Can you work these out from the drawing? Everything is in mm from the part's minimum corner. A direction names the side the tool comes from. Coordinates: 2 decimals unless noted, no trailing zeros. Loops run counter-clockwise (first coordinate to the right, second up) from the corner with the lowest first, then second, coordinate; pieces in that order, holes last.
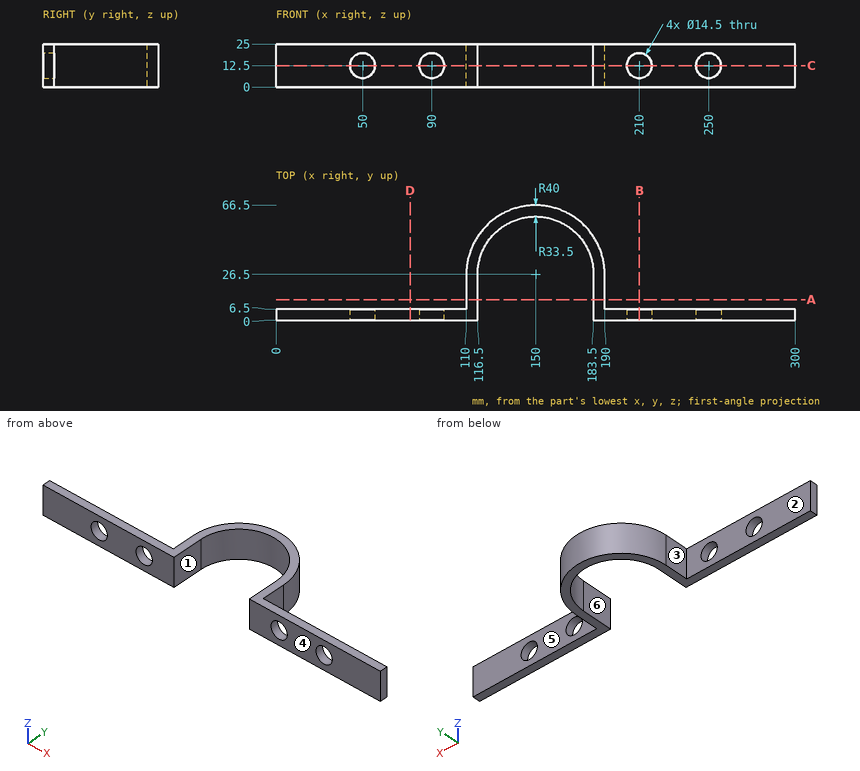
1. On a 3-axis mill with a long thin cutter (end or side, diameter ignored), from which of +Z, -Z, +X, -X, +Y, -Y can I reach the whole of each face in a straight line? I mean the marked faces 4, 5 and 6. Say none if no direction works.
2. I need wall thicknesses on line 1 along X through (y, z) = (5, 12.5); line 2 along Z through (x, y) = (250, 4); line 3 along X through (y, z) = (22, 17.75). Which ranges of each line are inside material? Lowest first, please.
3. I want a section at A-A (y = 12). Please give me the cut outline in (x, z).
4. I want a section at C-C (z = 12.5). Please give me the cut outline in (x, y).
5. We'd pull the mould along X, two halves only. Please class the marked faces 1, 2 and 3: +X half, -X half, draft (parallel to the pull), parting line (faces both ways), or undercut.
6. I want a section at D-D (x = 77.5). Please give me the cut outline in (y, z).
7. For pin 1 (6 mm diameter, centred on y = 19.5, z = 12.5, fed in from +X); pin 2 (7.5 mm diameter, centred on x = 63.5, z = 15, fed in from +Y); pin 3 (3 mm diameter, centred on y = 51, z = 21.5, fed in from -X), each with a flat end and sliding along its axis, tell me the tip position at first contact or that it passes through.
8. I want a section at B-B (x = 210). Please give me the cut outline in (y, z).
Response values:
1. face 4: +Z, -Z, +X, -X, -Y
1. face 5: +Z, -Z, +X, +Y
1. face 6: +Z, -Z, -Y
2. line 1: x = 0 to 42.75, 57.25 to 82.75, 97.25 to 116.5, 183.5 to 202.75, 217.25 to 242.75, 257.25 to 300
2. line 2: z = 0 to 5.25, 19.75 to 25
2. line 3: x = 110 to 116.5, 183.5 to 190
3. outline: (110, 0) - (116.5, 0) - (116.5, 25) - (110, 25) - close; (183.5, 0) - (190, 0) - (190, 25) - (183.5, 25) - close
4. outline: (0, 0) - (42.75, 0) - (42.75, 6.5) - (0, 6.5) - close; (57.25, 0) - (82.75, 0) - (82.75, 6.5) - (57.25, 6.5) - close; (97.25, 0) - (116.5, 0) - (116.5, 26.5) arc R33.5 cw to (183.5, 26.5) - (183.5, 0) - (202.75, 0) - (202.75, 6.5) - (190, 6.5) - (190, 26.5) arc R40 ccw to (110, 26.5) - (110, 6.5) - (97.25, 6.5) - close; (217.25, 0) - (242.75, 0) - (242.75, 6.5) - (217.25, 6.5) - close; (257.25, 0) - (300, 0) - (300, 6.5) - (257.25, 6.5) - close
5. face 1: undercut
5. face 2: draft
5. face 3: -X half
6. outline: (0, 0) - (6.5, 0) - (6.5, 25) - (0, 25) - close
7. pin 1: stops at x = 190
7. pin 2: stops at y = 6.5
7. pin 3: stops at x = 117.27
8. outline: (0, 0) - (6.5, 0) - (6.5, 5.25) - (0, 5.25) - close; (0, 19.75) - (6.5, 19.75) - (6.5, 25) - (0, 25) - close
